Work out the finished part from the listing and answer in its coordinate system (mm). Coordinates: 2 decimals unless noted, no trailing zeros. Order: outer loops, then holes, each group sorted by start corner. A loop starts at its lowest first (then second) coordinate and runs counter-clockwise, first axis right, second up. Notation, with made-up numbers: M 73.25,-31.5 L 116.25,-31.5 A18 cw 116.25,-3.5 Z; hole C 10.5,32.5 d4. An arc over 180 degrees is marked long. Write item = value, one per line. Start each with the question number.
Q1. Find section A-A on x = 75. Give the vertices of the cut face in (y, z).
Q2. Find section C-C on y = 8. Give the vertices of the cut face in (x, z).
Q3. Straight lines are drawn through the part: line 1 along Y through (x, z) = (6.35, 1.5) (3 decimals); line 2 along X through (y, z) = (7.5, 1.25) (3 decimals); line 3 along X through (y, z) = (5.75, 2.75). For each, find the intervals that lie inside material, in ascending order.
Q4. Find section B-B on z = 2.5. Give the number of separate pieces and of enclosed holes in the cut face, and give its area (3 significant figures).
Q5. This flat-tipped pin is pushed along its axis until it touches: P1, Ø5, axis at x = 6.35, y = 6.35, coming from the +Z side. Where does it stop, or does it pass through?
Q6. Find section D-D on x = 8. Give the vertices of the cut face in (y, z).
```python
from build123d import *

# Parameters (mm, degrees)
SKETCH2_W          = 82.55
SKETCH2_H          = 12.7
CRANK_HANDLE_DEPTH = 6.35
EDGE_1_R           = 6.35
EDGE_2_R           = 6.35
EDGE_3_R           = 6.35
EDGE_4_R           = 6.35
SKETCH3_R          = 3.175
HOLES_DEPTH        = 84.762252835


with BuildPart() as part:
    # Sketch2 → Crank Handle (new body)
    with BuildSketch(Plane.XY):
        with Locations((41.275, 6.35)):
            Rectangle(SKETCH2_W, SKETCH2_H)
    extrude(amount=CRANK_HANDLE_DEPTH)

    # Edge 1
    edge_1_edges = [part.edges().sort_by_distance(p)[0] for p in [
        (82.55, 12.7, 3.175),
    ]]
    fillet(edge_1_edges, radius=EDGE_1_R)

    # Edge 2
    edge_2_edges = [part.edges().sort_by_distance(p)[0] for p in [
        (82.55, 0, 3.175),
    ]]
    fillet(edge_2_edges, radius=EDGE_2_R - 0.0001)  # a hair under: the kernel refuses the full size

    # Edge 3
    edge_3_edges = [part.edges().sort_by_distance(p)[0] for p in [
        (0, 12.7, 3.175),
    ]]
    fillet(edge_3_edges, radius=EDGE_3_R)

    # Edge 4
    edge_4_edges = [part.edges().sort_by_distance(p)[0] for p in [
        (0, 0, 3.175),
    ]]
    fillet(edge_4_edges, radius=EDGE_4_R - 0.0001)  # a hair under: the kernel refuses the full size

    # Sketch3 → Holes (cut, through all)
    with BuildSketch(Plane.XY.offset(6.35)):
        with Locations((6.35, 6.35)):
            Circle(SKETCH3_R)
        with Locations((76.2, 6.35)):
            Circle(SKETCH3_R)
    extrude(amount=-HOLES_DEPTH, mode=Mode.SUBTRACT)


solid = part.part
```
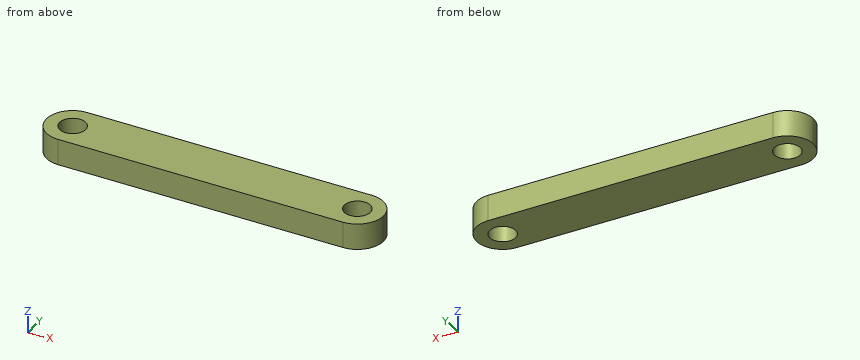
Findings below:
q1.outline = M 0,0 L 3.41,0 L 3.41,6.35 L 0,6.35 Z; M 9.29,0 L 12.7,0 L 12.7,6.35 L 9.29,6.35 Z
q2.outline = M 0.22,0 L 3.64,0 L 3.64,6.35 L 0.22,6.35 Z; M 9.06,0 L 73.49,0 L 73.49,6.35 L 9.06,6.35 Z; M 78.91,0 L 82.33,0 L 82.33,6.35 L 78.91,6.35 Z
q3.line_1 = 0 to 3.175, 9.525 to 12.7
q3.line_2 = 0.105 to 3.391, 9.309 to 73.241, 79.159 to 82.445
q3.line_3 = 0.03 to 3.23, 9.47 to 73.08, 79.32 to 82.52
q4.separate_pieces = 1
q4.enclosed_holes = 2
q4.area = 950 mm^2
q5.P1 = through
q6.outline = M 0,0 L 3.64,0 L 3.64,6.35 L 0,6.35 Z; M 9.06,0 L 12.7,0 L 12.7,6.35 L 9.06,6.35 Z
